from build123d import *

# Parameters (mm, degrees)
SKETCH_1_W                      = 25
SKETCH_1_H                      = 27
EXTRUDE_1_DEPTH                 = 3
CUT_EXTRUDE_1_REACH             = 38.919
SKETCH_2_R                      = 0.6
SKETCH_2_R_2                    = 12
CUT_EXTRUDE_1_DIRECTION_2_DEPTH = 37.918829884
EXTRUDE_2_DEPTH                 = 3
SKETCH_4_W                      = 24
SKETCH_4_H                      = 3
EXTRUDE_3_DEPTH                 = 20.9
EXTRUDE_3_DIRECTION_2_REACH     = 47.668
CUT_EXTRUDE_2_REACH             = 53.457
SKETCH_5_R                      = 0.6
CUT_EXTRUDE_2_DIRECTION_2_DEPTH = 52.456972317
CUT_EXTRUDE_4_DEPTH             = 3
EXTRUDE_4_DEPTH                 = 3


with BuildPart() as part:
    # Sketch 1 → Extrude 1 (new body)
    with BuildSketch(Plane.XY):
        with Locations((12.5, 13.5)):
            Rectangle(SKETCH_1_W, SKETCH_1_H)
    extrude(amount=EXTRUDE_1_DEPTH)

    # Sketch 2 → Cut-Extrude 1 (cut, up to next)
    with BuildSketch(Plane.XY.offset(3), mode=Mode.PRIVATE) as cut_extrude_1_sk1:
        with Locations(Location((2, 23.75, 0), (0, 0, 180))):
            Circle(SKETCH_2_R)
    cut_extrude_1_tool1 = extrude(cut_extrude_1_sk1.sketch, amount=-CUT_EXTRUDE_1_REACH, mode=Mode.PRIVATE) & part.part
    # Sketch 2 → Cut-Extrude 1 (cut, up to next)
    with BuildSketch(Plane.XY.offset(3), mode=Mode.PRIVATE) as cut_extrude_1_sk2:
        with Locations(Location((22.7, 23.75, 0), (0, 0, 180))):
            Circle(SKETCH_2_R)
    cut_extrude_1_tool2 = extrude(cut_extrude_1_sk2.sketch, amount=-CUT_EXTRUDE_1_REACH, mode=Mode.PRIVATE) & part.part
    # Sketch 2 → Cut-Extrude 1 (cut, up to next)
    with BuildSketch(Plane.XY.offset(3), mode=Mode.PRIVATE) as cut_extrude_1_sk3:
        with Locations(Location((22.7, 3.25, 0), (0, 0, 180))):
            Circle(SKETCH_2_R)
    cut_extrude_1_tool3 = extrude(cut_extrude_1_sk3.sketch, amount=-CUT_EXTRUDE_1_REACH, mode=Mode.PRIVATE) & part.part
    # Sketch 2 → Cut-Extrude 1 (cut, up to next)
    with BuildSketch(Plane.XY.offset(3), mode=Mode.PRIVATE) as cut_extrude_1_sk4:
        with Locations(Location((2, 3.25, 0), (0, 0, 180))):
            Circle(SKETCH_2_R)
    cut_extrude_1_tool4 = extrude(cut_extrude_1_sk4.sketch, amount=-CUT_EXTRUDE_1_REACH, mode=Mode.PRIVATE) & part.part
    # Sketch 2 → Cut-Extrude 1 (cut, up to next)
    with BuildSketch(Plane.XY.offset(3), mode=Mode.PRIVATE) as cut_extrude_1_sk5:
        with Locations((-6.3, 13.5)):
            Circle(SKETCH_2_R_2)
    cut_extrude_1_tool5 = extrude(cut_extrude_1_sk5.sketch, amount=-CUT_EXTRUDE_1_REACH, mode=Mode.PRIVATE) & part.part
    add(cut_extrude_1_tool1.solids().sort_by_distance((2, 23.75, 3))[0], mode=Mode.SUBTRACT)
    add(cut_extrude_1_tool2.solids().sort_by_distance((22.7, 23.75, 3))[0], mode=Mode.SUBTRACT)
    add(cut_extrude_1_tool3.solids().sort_by_distance((22.7, 3.25, 3))[0], mode=Mode.SUBTRACT)
    add(cut_extrude_1_tool4.solids().sort_by_distance((2, 3.25, 3))[0], mode=Mode.SUBTRACT)
    add(cut_extrude_1_tool5.solids().sort_by_distance((-6.3, 13.5, 3))[0], mode=Mode.SUBTRACT)

    # Sketch 2 → Cut-Extrude 1 direction 2 (cut)
    with BuildSketch(Plane.XY.offset(3)):
        with Locations(Location((2, 23.75, 0), (0, 0, 180))):
            Circle(SKETCH_2_R)
        with Locations(Location((22.7, 23.75, 0), (0, 0, 180))):
            Circle(SKETCH_2_R)
        with Locations(Location((22.7, 3.25, 0), (0, 0, 180))):
            Circle(SKETCH_2_R)
        with Locations(Location((2, 3.25, 0), (0, 0, 180))):
            Circle(SKETCH_2_R)
        with Locations((-6.3, 13.5)):
            Circle(SKETCH_2_R_2)
    extrude(amount=CUT_EXTRUDE_1_DIRECTION_2_DEPTH, mode=Mode.SUBTRACT)

    # Sketch 3 → Extrude 2 (add)
    with BuildSketch(Plane.XY.offset(3)):
        with BuildLine():
            ThreePointArc((0, 3.286773282), (-3.025761204, 1.955331953), (-6.3, 1.5))
            Line((-6.3, 1.5), (-6.3, -38.1))
            Line((-6.3, -38.1), (0, -38.1))
            Line((0, -38.1), (0, 0))
            Line((0, 0), (0, 3.286773282))
        make_face()
        with BuildLine():
            Line((-6.3, -38.1), (-6.3, 1.5))
            ThreePointArc((-6.3, 1.5), (-9.574238796, 1.955331953), (-12.6, 3.286773282))
            Line((-12.6, 3.286773282), (-12.6, -38.1))
            Line((-12.6, -38.1), (-6.3, -38.1))
        make_face()
    extrude(amount=-EXTRUDE_2_DEPTH)

    # Sketch 4 → Extrude 3 (add)
    with BuildSketch(Plane.XY.offset(3)):
        with Locations((-6.3, -1.5)):
            Rectangle(SKETCH_4_W, SKETCH_4_H)
    extrude_3 = extrude(amount=EXTRUDE_3_DEPTH)

    # Extrude 3 direction 2: up to this face of the body (flat: up to its plane)
    extrude_3_direction_2_end = Plane(part.part.faces().sort_by_distance((6.451782548, 13.5, 0))[0])
    # Sketch 4 → Extrude 3 direction 2 (add, up to the picked face)
    with BuildSketch(Plane.XY.offset(3), mode=Mode.PRIVATE) as extrude_3_direction_2_sk1:
        with Locations((-6.3, -1.5)):
            Rectangle(SKETCH_4_W, SKETCH_4_H)
    extrude_3_direction_2_tool1 = split(extrude(extrude_3_direction_2_sk1.sketch, amount=-EXTRUDE_3_DIRECTION_2_REACH, mode=Mode.PRIVATE), bisect_by=extrude_3_direction_2_end, keep=Keep.BOTH, mode=Mode.PRIVATE)
    extrude_3_direction_2 = extrude_3_direction_2_tool1.solids().sort_by(Axis((-6.3, -1.5, 3), (0, 0, -1)))[0]
    add(extrude_3_direction_2)

    # Sketch 5 → Cut-Extrude 2 (cut, up to next)
    with BuildSketch(Plane(origin=(0, 0, 0), x_dir=(1, 0, 0), z_dir=(0, 1, 0)), mode=Mode.PRIVATE) as cut_extrude_2_sk1:
        with Locations(Location((-16.55, -21.5, 0), (0, 0, 90))):
            Circle(SKETCH_5_R)
    cut_extrude_2_tool1 = extrude(cut_extrude_2_sk1.sketch, amount=-CUT_EXTRUDE_2_REACH, mode=Mode.PRIVATE) & part.part
    # Sketch 5 → Cut-Extrude 2 (cut, up to next)
    with BuildSketch(Plane(origin=(0, 0, 0), x_dir=(1, 0, 0), z_dir=(0, 1, 0)), mode=Mode.PRIVATE) as cut_extrude_2_sk2:
        with Locations(Location((3.95, -21.5, 0), (0, 0, 90))):
            Circle(SKETCH_5_R)
    cut_extrude_2_tool2 = extrude(cut_extrude_2_sk2.sketch, amount=-CUT_EXTRUDE_2_REACH, mode=Mode.PRIVATE) & part.part
    cut_extrude_2_1 = cut_extrude_2_tool1.solids().sort_by_distance((-16.55, 0, 21.5))[0]
    add(cut_extrude_2_1, mode=Mode.SUBTRACT)
    cut_extrude_2_2 = cut_extrude_2_tool2.solids().sort_by_distance((3.95, 0, 21.5))[0]
    add(cut_extrude_2_2, mode=Mode.SUBTRACT)
    cut_extrude_2 = cut_extrude_2_1 + cut_extrude_2_2  # Cut-Extrude 2 as one shape, for the pattern or mirror that repeats it

    # Sketch 5 → Cut-Extrude 2 direction 2 (cut)
    with BuildSketch(Plane(origin=(0, 0, 0), x_dir=(1, 0, 0), z_dir=(0, 1, 0))):
        with Locations(Location((-16.55, -21.5, 0), (0, 0, 90))):
            Circle(SKETCH_5_R)
        with Locations(Location((3.95, -21.5, 0), (0, 0, 90))):
            Circle(SKETCH_5_R)
    cut_extrude_2_direction_2 = extrude(amount=CUT_EXTRUDE_2_DIRECTION_2_DEPTH, mode=Mode.SUBTRACT)

    # Mirror 3: Extrude 3, Extrude 3 direction 2, Cut-Extrude 2, Cut-Extrude 2 direction 2 across plane
    add(extrude_3.mirror(Plane(origin=(0, -19.05, 0), x_dir=(0, 0, 1), z_dir=(0, -1, 0))))
    add(extrude_3_direction_2.mirror(Plane(origin=(0, -19.05, 0), x_dir=(0, 0, 1), z_dir=(0, -1, 0))))
    add(cut_extrude_2.mirror(Plane(origin=(0, -19.05, 0), x_dir=(0, 0, 1), z_dir=(0, -1, 0))), mode=Mode.SUBTRACT)
    add(cut_extrude_2_direction_2.mirror(Plane(origin=(0, -19.05, 0), x_dir=(0, 0, 1), z_dir=(0, -1, 0))), mode=Mode.SUBTRACT)

    # Sketch 9 → Cut-Extrude 4 (cut)
    with BuildSketch(Plane.XZ.offset(38.1)):
        with BuildLine():
            ThreePointArc((-8.851470164, 23.9), (-11.965615436, 22.628722169), (-14.55, 20.475816105))
            ThreePointArc((-14.55, 20.475816105), (-10.189087297, 2.910442186), (4.7, 13.2))
            ThreePointArc((4.7, 13.2), (3.989557814, 17.089087297), (1.95, 20.475816105))
            ThreePointArc((1.95, 20.475816105), (-0.634384564, 22.628722169), (-3.748529836, 23.9))
            Line((-3.748529836, 23.9), (-8.851470164, 23.9))
        make_face()
        with BuildLine():
            ThreePointArc((-3.748529836, 23.9), (-6.3, 24.2), (-8.851470164, 23.9))
            Line((-8.851470164, 23.9), (-3.748529836, 23.9))
        make_face()
        with BuildLine():
            Line((-8.851470164, 23.9), (-14.55, 23.9))
            Line((-14.55, 23.9), (-14.55, 20.475816105))
            ThreePointArc((-14.55, 20.475816105), (-11.965615436, 22.628722169), (-8.851470164, 23.9))
        make_face()
        with BuildLine():
            Line((1.95, 23.9), (-3.748529836, 23.9))
            ThreePointArc((-3.748529836, 23.9), (-0.634384564, 22.628722169), (1.95, 20.475816105))
            Line((1.95, 20.475816105), (1.95, 23.9))
        make_face()
    extrude(amount=-CUT_EXTRUDE_4_DEPTH, mode=Mode.SUBTRACT)

    # Sketch 10 → Extrude 4 (add)
    with BuildSketch(Plane.XZ.offset(38.1)):
        with BuildLine():
            ThreePointArc((-18.3, 23.9), (-22.377624203, 13.2), (-18.3, 2.5))
            Line((-18.3, 2.5), (-18.3, 23.9))
        make_face()
        with BuildLine():
            Line((5.7, 23.9), (5.7, 2.5))
            ThreePointArc((5.7, 2.5), (8.723672827, 7.474682997), (9.777624203, 13.2))
            ThreePointArc((9.777624203, 13.2), (8.723672827, 18.925317003), (5.7, 23.9))
        make_face()
    extrude(amount=-EXTRUDE_4_DEPTH)


solid = part.part
Check sheet for the modelled part. Datum: model origin and axes. Units: mm. A direction names the side the tool comes from. Give positions to 0.01 mm unless a question says otherwise; leave off trailing zeros. Write each loop counter-clockwise with the first axis right and the second up, starting at its lowest first coordinate (ties: lowest second). Pieces come first, ordered by that corner, then holes. Notation, with made-up numbers: (-0.75, 70) -> (58.25, 70) arc R10 ccw to (58.25, 82) -> close; hole circle Ø10 at (-28.5, 71.25). An arc over 180 degrees is marked (long way). One line per item, written item: value. Start each with the question number.
Item 1: Tool access check on faces 1 (the flat face through (-14.55, -37, 22)), 2 (the flat face through (5.7, -37, 1)), 3 (the flat face through (-12.6, -19, 2)), 4 (the flat face through (0, 25, 1)). Record the directions out of +Z, -Z, +X, -X, +Y, -Y that give a thin tool (end or side, any length) a straight path to the whole face; none if there is none.
Item 2: Section check D-D on z = 15.5. Record the cut outline in (x, y), then the cut area to 3 significant figures.
Item 3: Draft check along Y on faces 5 (the flat face through (-12.6, 2, 2)), 6 (the flat face through (-6, -19, 3)), 7 (the flat face through (12, 27, 1)). Enter one of: +Y half, -Y half, draft (parallel to the pull), parting line (faces both ways), or undercut.
Item 4: Gauge pin test, flat ends, axial feed: pin 1 (12 mm diameter, centred on x = 2, z = 18, fed in from +Y); pin 2 (10 mm diameter, centred on y = -0.5, z = 20.5, fed in from +X); pin 3 (3 mm diameter, centred on x = -8, z = 8.5, fed in from -Y). Record the tip position at first contact, or that the pin passes through.
Item 5: Material ranges on probe 1 along Y at (x, z) = (22.7, 0.9); probe 2 along X at (y, z) = (23.75, 1.25); probe 3 along X at (y, z) = (-0.7, 21.5), recorded low to high. Write a range as from..to.
Item 6: Section check A-A on z = 7.5. Record the cut outline in (x, y), then the cut area to 3 significant figures.
Item 7: Section check C-C on y = -7. Record the cut outline in (x, z), then the cut area to 3 significant figures.
Item 8: Section check B-B on x = -8.5. Record the cut outline in (y, z), then the cut area to 3 significant figures.
Results list:
1. face 1: +Z, -Y
1. face 2: -Z, +X, -Y
1. face 3: +Z, -Z, -X
1. face 4: +Z, -Z, -X, +Y
2. outline: (-22.21, -38.1) -> (-17.06, -38.1) -> (-17.06, -35.1) -> (-22.21, -35.1) -> close; (-18.3, -3) -> (5.7, -3) -> (5.7, 0) -> (-18.3, 0) -> close; (4.46, -38.1) -> (9.61, -38.1) -> (9.61, -35.1) -> (4.46, -35.1) -> close
2. area: 103 mm²
3. face 5: draft
3. face 6: undercut
3. face 7: +Y half
4. pin 1: y = 0
4. pin 2: x = 5.7
4. pin 3: y = -3
5. probe 1: 0..2.65, 3.85..23.15, 24.35..27
5. probe 2: 0..1.4, 2.6..22.1, 23.3..25
5. probe 3: -18.3..-17.15, -15.95..3.35, 4.55..5.7
6. outline: (-21.33, -38.1) -> (-15.71, -38.1) -> (-15.71, -35.1) -> (-21.33, -35.1) -> close; (-18.3, -3) -> (5.7, -3) -> (5.7, 0) -> (-18.3, 0) -> close; (3.11, -38.1) -> (8.73, -38.1) -> (8.73, -35.1) -> (3.11, -35.1) -> close
6. area: 106 mm²
7. outline: (-12.6, 0) -> (0, 0) -> (0, 3) -> (-12.6, 3) -> close
7. area: 37.8 mm²
8. outline: (-38.1, 0) -> (1.7, 0) -> (1.7, 3) -> (0, 3) -> (0, 23.9) -> (-3, 23.9) -> (-3, 3) -> (-35.1, 3) -> (-35.1, 2.42) -> (-38.1, 2.42) -> close
8. area: 180 mm²
